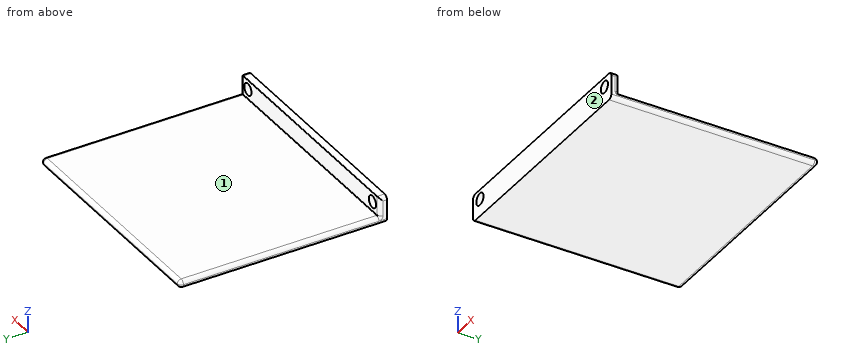
from build123d import *

# Parameters (mm, degrees)
SKETCH1_W           = 60
SKETCH1_H           = 54
BOSS_EXTRUDE1_DEPTH = 2
SKETCH2_W           = 60
SKETCH2_H           = 2
BOSS_EXTRUDE2_DEPTH = 5
SKETCH3_R           = 1.56
CUT_EXTRUDE1_DEPTH  = 5
FILLET1_R           = 0.1
FILLET2_R           = 1
FILLET3_R           = 0.1


with BuildPart() as part:
    # Sketch1 → Boss-Extrude1 (new body)
    with BuildSketch(Plane.XY):
        Rectangle(SKETCH1_W, SKETCH1_H)
    extrude(amount=BOSS_EXTRUDE1_DEPTH)

    # Sketch2 → Boss-Extrude2 (add)
    with BuildSketch(Plane.XY.offset(2)):
        with Locations((0, -26)):
            Rectangle(SKETCH2_W, SKETCH2_H)
    extrude(amount=BOSS_EXTRUDE2_DEPTH)

    # Sketch3 → Cut-Extrude1 (cut)
    with BuildSketch(Plane(origin=(0, -25, 0), x_dir=(1, 0, 0), z_dir=(0, 1, 0))):
        with Locations(Location((27, -4.5, 0), (0, 0, 270))):
            Circle(SKETCH3_R)
        with Locations(Location((-27, -4.5, 0), (0, 0, 270))):
            Circle(SKETCH3_R)
    extrude(amount=-CUT_EXTRUDE1_DEPTH, mode=Mode.SUBTRACT)

    # Fillet1
    fillet1_edges = [part.edges().sort_by_distance(p)[0] for p in [
        (0, -25, 2),
    ]]
    fillet(fillet1_edges, radius=FILLET1_R)

    # Fillet2
    fillet2_edges = [part.edges().sort_by_distance(p)[0] for p in [
        (-30, 1.05, 2),
        (-30, -25, 4.55),
        (30, -25, 4.55),
        (-30, -26, 7),
        (30, -26, 7),
        (30, 1.05, 2),
        (-30, -24.970710678, 2.029289322),
        (30, -24.970710678, 2.029289322),
        (-30, 0, 0),
        (0, 27, 0),
        (30, 0, 0),
        (-30, 27, 1),
        (30, 27, 1),
        (0, 27, 2),
    ]]
    fillet(fillet2_edges, radius=FILLET2_R - 0.0001)  # a hair under: the kernel refuses the full size

    # Fillet3
    fillet3_edges = [part.edges().sort_by_distance(p)[0] for p in [
        (0, -25, 7),
        (-29.763319687, -25.353915697, 6.646084303),
        (29.763319687, -25.353915697, 6.646084303),
    ]]
    fillet(fillet3_edges, radius=FILLET3_R)


solid = part.part
The model under review builds one solid part; all positions refer to its coordinate system, in mm. Face numbers are marked on the shaded views. A direction names the side the tool comes from. Give positions to 0.01 mm unless a question says otherwise; leave off trailing zeros. Order: outer loops, then holes, each group sorted by start corner. A loop starts at its lowest first (then second) coordinate and runs counter-clockwise, first axis right, second up. Notation, with made-up numbers: M 24,57.5 L 30,57.5 A27 cw 30,91.5 Z; hole C 57,-34.75 d10. An arc over 180 degrees is marked long. One line per question, with ' | ' between items. Start each with the question number.
1) Consider section B-B, the plane z = 4.5. Give the boundary of the cut face in (x, y), then the cut area to 3 significant figures.
2) For the marked faces 1 and 2, list the 3-axis set-ups (+Z, -Z, +X, -X, +Y, -Y) from which the entire face can be reached by the end or side of a thin tool; tool diameter is ignored.
3) Wall thickness on L1, parallel to X at y = -26.25, z = 4.5; L2, parallel to Y at x = -14, z = 3.75; L3, parallel to Z at x = -20, y = 4.5: over which ranges is each line inside the solid? List them lowest first. Write a range as from..to.
4) Clearance check with flat-ended pins moving along their axes: P1, Ø10, axis at x = 13.5, y = 0, coming from the +Z side; P2, Ø2.5, axis at x = 27, z = 4.5, coming from the +Y side; P3, Ø2.5, axis at x = 5.5, z = 3.5, coming from the +Y side; P4, Ø3, axis at y = 18, z = 3, coming from the -X side. State where each tip first meets the part, or that it passes through.
Found:
1) outline: M -30,-27 L -28.56,-27 L -28.56,-25 L -29,-25 A1 ccw -30,-26 Z; M -25.44,-27 L 25.44,-27 L 25.44,-25 L -25.44,-25 Z; M 28.56,-27 L 30,-27 L 30,-26 A1 ccw 29,-25 L 28.56,-25 Z | area: 107 mm²
2) face 1: +Z, +X, -X, +Y | face 2: +Z, -Z, +X, -X, -Y
3) L1: x = -30..-28.56, -25.44..25.44, 28.56..30 | L2: y = -27..-25 | L3: z = 0..2
4) P1: stops at z = 2 | P2: passes through | P3: stops at y = -25 | P4: stops at x = -29.87
